Autodesk Inventor part; units mm, degrees
ref_plane "YZ Plane" through (0, 0, 0) normal (1, 0, 0) x (0, 1, 0)
ref_plane "XZ Plane" through (0, 0, 0) normal (0, 1, 0) x (-1, 0, 0)
ref_plane "XY Plane" through (0, 0, 0) normal (0, 0, 1) x (1, 0, 0)
sketch "スケッチ1" plane through (0, 0, 0) normal (0, 1, 0) x (-1, 0, 0)
  line L0 (0, 0) -> (33, 0)
  line L1 (33, 0) -> (33, -38.3)
  line L2 (33, -38.3) -> (0, -38.3)
  line L3 (0, -38.3) -> (0, 0)
  dimension "d0" = 33
  dimension "d1" = 38.3
extrude "押し出し1" add sketch "スケッチ1" along normal blind 20.2
sketch "スケッチ2" plane through (0, 20.2, 0) normal (0, 1, 0) x (1, 0, 0)
  line L0 (-33, 38.3) -> (-33, 0)
  line L1 (-33, 19.15) -> (0, 19.15)
  line L2 (0, 0) -> (0, 38.3)
  point P0 (-27.7, 19.15)
  point P1 (-5.3, 19.15)
  dimension "d4" = 5.3
  dimension "d5" = 5.3
sketch "スケッチ3" plane through (0, 20.2, 0) normal (0, 1, 0) x (1, 0, 0)
  point P0 (0, 0)
sketch "スケッチ4" plane through (0, 20.2, 0) normal (0, 1, 0) x (1, 0, 0)
  circle A0 centre (-5.3, 19.15) radius 4.3
  circle A1 centre (-27.7, 19.15) radius 4.3
  point P0 (0, 0)
  dimension "d6" = 8.6
  dimension "d7" = 8.6
hole "穴1" at (-5.3, 20.2, -19.15) direction (0, -1, 0) diameter 8.6 end through all
hole "穴2" at (-27.7, 20.2, -19.15) direction (0, -1, 0) diameter 8.6 end through all
sketch "スケッチ5" plane through (-33, 0, 0) normal (0, 0, 1) x (1, 0, 0)
  line L0 (33, 20.2) -> (0, 20.2)
  line L1 (16.5, 20.2) -> (16.5, 0)
  circle A0 centre (16.5, 10.1) radius 5
  circle A1 centre (16.5, 10.1) radius 3.1
  point P0 (33, 0)
  dimension "d22" = 10
  dimension "d23" = 6.2
sketch "スケッチ6" plane through (0, 0, 0) normal (1, 0, 0) x (0, 0, -1)
  line L0 (0, 0) -> (38.3, 0)
  line L1 (12.25, 0) -> (12.25, 20.2)
  line L2 (0, 20.2) -> (38.3, 20.2)
  line L3 (25.25, 0) -> (25.25, 20.2)
  point P0 (12.25, 9.5)
  point P1 (25.25, 11.7)
  dimension "d26" = 9.5
  dimension "d27" = 8.5
sketch "スケッチ7" plane through (0, 0, 0) normal (1, 0, 0) x (0, 0, -1)
  point P0 (0, 0)
hole "穴3" at (0, 9.5, -12.25) at (0, 11.7, -25.25) direction (-1, 0, 0) diameter 3.1 depth 6 tip angle 118
extrude "押し出し3" add sketch "スケッチ5" along normal blind 1 contours A0 L1 A1 | L1 A1 A0
sketch "スケッチ8" plane through (-33, 0, 0) normal (0, 0, 1) x (1, 0, 0)
  line L0 (0, 20.2) -> (33, 20.2)
  line L1 (16.5, 20.2) -> (16.5, 0)
  line L2 (33, 0) -> (0, 0)
  point P0 (16.5, 10.1)
hole "穴4" at (-16.5, 10.1, 0) direction (0, 0, -1) diameter 6.2 depth 10
properties part number "コガネイ_BDA16x5"
Work out the finished part from the listing and answer in its coordinate system (mm). A direction names the side the tool comes from. Give positions to 0.01 mm unless a question says otherwise; leave off trailing zeros. Write each loop counter-clockwise with the first axis right and the second up, starting at its lowest first coordinate (ties: lowest second). Pieces come first, ordered by that corner, then holes. Notation, with made-up numbers: (11.5, 41.25) - (37.5, 41.25) arc R28 ccw to (37.5, 79.25) - close; hole circle Ø3 at (13, 65.5). An arc over 180 degrees is marked (long way). One line per item, written item: value. Start each with the question number.
1. Find section C-C (z = -8). Write down the section's boundary in (x, y).
2. Given pin 1 (1.5 mm diameter, centred on x = -9.5, y = 7.5, fed in from +Z); pin 2 (1.9 mm diameter, centred on x = -16, y = 9.5, fed in from +Z), each flat-ended and moving along its own axis, determine where each tip first touches the part or whether it passes through.
3. Find section A-A (x = -5.3). Write down the section's boundary in (y, z).
4. For a pull along Z with two mould halves and no side action, classify faces 4 (the cylindrical face through (-17.58, 14.98, 0.49)), 5 (the conical face through (-6.77, 9.68, -12.05)), 6 (the flat face through (-19, 8, 1)) as +Z half, -Z half, draft (parallel to the pull), parting line (faces both ways), or undercut.
5. For faces 1 (the flat face through (-17, 10, -10)), 2 (the flat face through (0, 10, -19)), 3 (the cylindrical face through (-3.04, 10.44, -11.02)), determine the directions among +Z, -Z, +X, -X, +Y, -Y from which every point of the face is accessible in a straight line to the end or side of a thin tool.
6. Find section D-D (y = 14.5). Write down the section's boundary in (x, z), then the cut area to 3 significant figures.
7. Find section B-B (z = -19.15). Write down the section's boundary in (x, y), then the cut area to 3 significant figures.
8. Consider probe 1 along X at (y, z) = (11.25, -19); probe 2 along Y at (x, z) = (-16.5, -4); probe 3 along X at (y, z) = (10.1, -4.5). Determine where each line is inside the solid, lowest interval first.
Geometry results:
1. outline: (-33, 0) - (0, 0) - (0, 20.2) - (-33, 20.2) - close; hole circle Ø6.2 at (-16.5, 10.1)
2. pin 1: z = 0
2. pin 2: z = -10
3. outline: (0, -38.3) - (20.2, -38.3) - (20.2, -23.45) - (0, -23.45) - close; (0, -14.85) - (20.2, -14.85) - (20.2, 0) - (0, 0) - close; hole circle Ø3.1 at (9.5, -12.25); hole circle Ø3.1 at (11.7, -25.25)
4. face 4: draft
4. face 5: undercut
4. face 6: +Z half
5. face 1: +Z
5. face 2: +Z, -Z, +X, +Y, -Y
5. face 3: +X
6. outline: (-33, -38.3) - (0, -38.3) - (0, 0) - (-14.13, 0) - (-14.13, 1) - (-18.87, 1) - (-18.87, 0) - (-33, 0) - close; hole circle Ø8.6 at (-27.7, -19.15); hole circle Ø8.6 at (-5.3, -19.15)
6. area: 1,150 mm2
7. outline: (-33, 0) - (-32, 0) - (-32, 20.2) - (-33, 20.2) - close; (-23.4, 0) - (-9.6, 0) - (-9.6, 20.2) - (-23.4, 20.2) - close; (-1, 0) - (0, 0) - (0, 20.2) - (-1, 20.2) - close
7. area: 319 mm2
8. probe 1: -33 to -32, -23.4 to -9.6, -1 to 0
8. probe 2: 0 to 7, 13.2 to 20.2
8. probe 3: -33 to -19.6, -13.4 to 0
